Verification items for the finished model (mm, model axes). A direction names the side the tool comes from. Coordinates: 2 decimals unless noted, no trailing zeros. Order: outer loops, then holes, each group sorted by start corner. A loop starts at its lowest first (then second) coordinate and runs counter-clockwise, first axis right, second up. Notation, with made-up numbers: (38.5, 69.25) -> (96.5, 69.25) arc R11 ccw to (96.5, 78.25) -> close; hole circle Ø10 at (43.25, -7.75). An arc over 180 degrees is marked (long way). Write item = value, one per line. Start each with the question number.
1. Release check for a two-part mould opening along X. For faces 1 (the cylindrical face through (-32.175, 0.986, 94.616)), 2 (the flat face through (-33, 2, 0)), 3 (the flat face through (-26.65, 2.46, 97.59)) record: +X half, -X half, draft (parallel to the pull), parting line (faces both ways), or undercut.
2. Thickness scan on line 1 along X through (y, z) = (1.35, 5.08); line 2 along Z through (x, y) = (-5, 3.3); line 3 along X through (y, z) = (3.1, 120). Record the ranges inside material, lowest first. Write a range as from..to.
3. Set-up check for faces 4 (the flat face through (-67.7, 2, 24)), 5 (the flat face through (0, 2, 34)), 6 (the flat face through (-7, 2, 63)): record each of +Z, -Z, +X, -X, +Y, -Y from which the full face is reachable in a straight line by a thin tool's end or side.
4. Cross-section at D-D on z = 63.08. Record the cut outline in (x, y), plus the area to 3 significant figures.
5. Cross-section at A-A on z = 5.08. Record the cut outline in (x, y), plus the area to 4 significant figures.
6. Cross-section at C-C on x = -5.08. Record the cut outline in (y, z), plus the area to 3 significant figures.
7. Cross-section at B-B on x = -62.62. Record the cut outline in (y, z).
8. Go/stop test with flat-tipped pins: P1, Ø2.5, axis at y = 3, z = 12.5, coming from the -X side; P2, Ø9.5, axis at x = -5.08, z = 63.08, coming from the +Y side; P3, Ø1.8, axis at x = -4, z = 5, coming from the +Y side; P4, Ø1.5, axis at x = -89, y = 2, coming from the -Z side. Record where each tip stops, or that it passes through.
from build123d import *

# Parameters (mm, degrees)
BOSS_EXTRUDE1_DEPTH   = 5
F_4_0MM_DOWEL_HOLE1_D = 3.5
SKETCH4_R             = 3
CUT_EXTRUDE1_DEPTH    = 3


with BuildPart() as part:
    # Sketch1 → Boss-Extrude1 (new body)
    with BuildSketch(Plane(origin=(0, 0, 0), x_dir=(1, 0, 0), z_dir=(0, 1, 0))):
        Polygon((0, 0), (-67.7, 0), (-67.7, -48.64), (-104.14, -48.64), (-104.140084457, -126.999681711), (-52.560084457, -126.999681711), (0, -67.34), align=None)
    extrude(amount=BOSS_EXTRUDE1_DEPTH)

    # Ø4.0mm Dowel Hole1 (through all)
    with Locations(Plane(origin=(-99.060084457, 5, 121.919681711), x_dir=(0, 0, 1), z_dir=(0, 1, 0))):
        with Locations((0, 0), (0, 43.21), (-58.839681711, 93.980084457), (-27.682634748, 68.593581655), (-116.839681711, 93.980084457), (-116.839681711, 36.440084457)):
            Hole(F_4_0MM_DOWEL_HOLE1_D / 2)

    # Sketch4 → Cut-Extrude1 (cut)
    with BuildSketch(Plane(origin=(0, 5, 0), x_dir=(1, 0, 0), z_dir=(0, 1, 0))):
        with Locations(Location((-99.060084457, -121.919681711, 0), (0, 0, 270))):
            Circle(SKETCH4_R)
        with Locations(Location((-55.850084457, -121.919681711, 0), (0, 0, 270))):
            Circle(SKETCH4_R)
        with Locations(Location((-30.466502802, -94.237046963, 0), (0, 0, 270))):
            Circle(SKETCH4_R)
        with Locations(Location((-5.08, -63.08, 0), (0, 0, 270))):
            Circle(SKETCH4_R)
        with Locations(Location((-5.08, -5.08, 0), (0, 0, 270))):
            Circle(SKETCH4_R)
        with Locations(Location((-62.62, -5.08, 0), (0, 0, 270))):
            Circle(SKETCH4_R)
    extrude(amount=-CUT_EXTRUDE1_DEPTH, mode=Mode.SUBTRACT)


solid = part.part
Worked out:
q1.face_1 = undercut
q1.face_2 = draft
q1.face_3 = +X half
q2.line_1 = -67.7..-64.37, -60.87..-6.83, -3.33..0
q2.line_2 = 0..2.08, 8.08..60.08, 66.08..73.02
q2.line_3 = -104.14..-101.37, -96.75..-58.16, -53.54..-46.39
q3.face_4 = -Z, -X, +Y, -Y
q3.face_5 = +Z, -Z, +X, +Y, -Y
q3.face_6 = +Y
q4.outline = (-104.14, 0) -> (-6.83, 0) -> (-6.83, 2) -> (-8.08, 2) -> (-8.08, 5) -> (-104.14, 5) -> close; (-3.33, 0) -> (0, 0) -> (0, 5) -> (-2.08, 5) -> (-2.08, 2) -> (-3.33, 2) -> close
q4.area = 496 mm²
q5.outline = (-67.7, 0) -> (-64.37, 0) -> (-64.37, 2) -> (-65.62, 2) -> (-65.62, 5) -> (-67.7, 5) -> close; (-60.87, 0) -> (-6.83, 0) -> (-6.83, 2) -> (-8.08, 2) -> (-8.08, 5) -> (-59.62, 5) -> (-59.62, 2) -> (-60.87, 2) -> close; (-3.33, 0) -> (0, 0) -> (0, 5) -> (-2.08, 5) -> (-2.08, 2) -> (-3.33, 2) -> close
q5.area = 288.5 mm²
q6.outline = (0, 0) -> (5, 0) -> (5, 2.08) -> (2, 2.08) -> (2, 3.33) -> (0, 3.33) -> close; (0, 6.83) -> (2, 6.83) -> (2, 8.08) -> (5, 8.08) -> (5, 60.08) -> (2, 60.08) -> (2, 61.33) -> (0, 61.33) -> close; (0, 64.83) -> (2, 64.83) -> (2, 66.08) -> (5, 66.08) -> (5, 73.11) -> (0, 73.11) -> close
q6.area = 316 mm²
q7.outline = (0, 0) -> (5, 0) -> (5, 2.08) -> (2, 2.08) -> (2, 3.33) -> (0, 3.33) -> close; (0, 6.83) -> (2, 6.83) -> (2, 8.08) -> (5, 8.08) -> (5, 127) -> (0, 127) -> close
q8.P1 = -67.7
q8.P2 = 5
q8.P3 = 2
q8.P4 = 48.64
